Could you check a few things on this model? Use its own coordinates, in mm. A direction names the side the tool comes from. Give positions to 0.01 mm unless a question says otherwise; leave off trailing zeros. Write each loop counter-clockwise with the first axis right and the second up, starting at its lowest first coordinate (ties: lowest second). Pieces come first, ordered by that corner, then holes. Notation, with made-up numbers: M 15,-24 L 71,-24 A26 ccw 71,8 Z; hole C 83.5,2.5 d11. An arc over 180 degrees is marked long. Answer as CSV lines item,"result". Start each with the question number.
from build123d import *

# Parameters (mm, degrees)
F0_R     = 6.985
F0_R_2   = 1.804442
F0_R_3   = 1.4986
F0_R_4   = 1.27
F0_R_5   = 0.4445
F0_R_6   = 1.5
F1_DEPTH = 3.175


with BuildPart() as f1:
    # F0 (on Top) → F1 (new body)
    with BuildSketch(Plane.XY):
        with BuildLine():
            ThreePointArc((-31.595516, -60.452), (-29.735644, -64.942128), (-25.245516, -66.802))
            Line((-25.245516, -66.802), (38.254484, -66.802))
            ThreePointArc((38.254484, -66.802), (42.744612, -64.942128), (44.604484, -60.452))
            Line((44.604484, -60.452), (44.604484, 15.748))
            ThreePointArc((44.604484, 15.748), (42.744612, 20.238128), (38.254484, 22.098))
            Line((38.254484, 22.098), (0.154484, 22.098))
            ThreePointArc((0.154484, 22.098), (-4.335644, 20.238128), (-6.195516, 15.748))
            Line((-6.195516, 15.748), (-6.195516, -16.002))
            ThreePointArc((-6.195516, -16.002), (-8.055388, -20.492128), (-12.545516, -22.352))
            Line((-12.545516, -22.352), (-25.245516, -22.352))
            ThreePointArc((-25.245516, -22.352), (-29.735644, -24.211872), (-31.595516, -28.702))
            Line((-31.595516, -28.702), (-31.595516, -60.452))
        make_face()
        with Locations((-13.307516, -46.1518)):
            Circle(F0_R, mode=Mode.SUBTRACT)
        with Locations((4.801642, -53.465958)):
            Circle(F0_R_2, mode=Mode.SUBTRACT)
        with Locations((34.114284, -53.784222)):
            Circle(F0_R_3, mode=Mode.SUBTRACT)
        with Locations((35.079484, -46.1518)):
            Circle(F0_R_4, mode=Mode.SUBTRACT)
        with Locations((4.496019, 15.415596)):
            Circle(F0_R_5, mode=Mode.SUBTRACT)
        with Locations((8.790484, 0)):
            Circle(F0_R_4, mode=Mode.SUBTRACT)
        with Locations((6.604484, 13.1064)):
            Circle(F0_R_3, mode=Mode.SUBTRACT)
        with Locations((35.604484, 13.1064)):
            Circle(F0_R_6, mode=Mode.SUBTRACT)
    extrude(amount=F1_DEPTH)


solid = f1.part
1. Thinking about a two-plate mould opening in X: for faces 3 (the flat face through (14, -22, 0)), 4 (the cylindrical face through (42.695, -64.991, 1.565)), 5 (the cylindrical face through (-29.785, -64.892, 1.565)), 6 (the cylindrical face through (9.96, -0.49, 1.57)), which applies, pulls with the +X half, pulls with the -X half, needs draft (parallel to the pull), parting line crosses it, or undercut?
2. Imagine slicing it at A-A, the plane y = 0. Please give me the cut outline in (x, z) (3 decimals), plus the area to 3 significant figures.
3. Imagine slicing it at B-B, the plane z = 1.1. State how many separate pieces and enclosed holes the cut face has, plus the area to 3 significant figures.
4. On a 3-axis mill with a long thin cutter (end or side, diameter ignored), from which of +Z, -Z, +X, -X, +Y, -Y can I reach the whole of each face in a straight line? I mean faces 1 (the cylindrical face through (34.5, 14.12, 1.57)), 2 (the flat face through (-6.196, 0, 2)). Say none if no direction works.
5. Imagine slicing it at C-C, the plane x = -21.5. Please give me the cut outline in (y, z) (3 decimals).
6. Please list where these lines run through material, in increasing order: line 1 (Y direction, x = -13.5, z = 2); line 2 (Y direction, x = 6, z = 2.85); line 3 (Y direction, x = -23.5, z = 0.9).
Solutions:
1,face 3,"needs draft"
1,face 4,"pulls with the +X half"
1,face 5,"pulls with the -X half"
1,face 6,"undercut"
2,outline,"M -6.196,0 L 7.52,0 L 7.52,3.175 L -6.196,3.175 Z; M 10.06,0 L 44.604,0 L 44.604,3.175 L 10.06,3.175 Z"
2,area,"153 mm²"
3,separate pieces,"1"
3,enclosed holes,"8"
3,area,"5,420 mm²"
4,face 1,"+Z, -Z"
4,face 2,"+Z, -Z, -X, +Y"
5,outline,"M -66.802,0 L -22.352,0 L -22.352,3.175 L -66.802,3.175 Z"
6,line 1,"-66.8 to -53.13, -39.17 to -22.35"
6,line 2,"-66.8 to -54.82, -52.12 to 11.74, 14.48 to 22.1"
6,line 3,"-66.8 to -22.35"
